Here's how the part is built. I have some questions about the finished solid (model axes, mm). Face numbers are marked on the shaded views. A direction names the side the tool comes from. Round coordinates to 2 decimals unless told otherwise and drop trailing zeros. Loops run counter-clockwise (first coordinate to the right, second up) from the corner with the lowest first, then second, coordinate; pieces in that order, holes last. Notation, with made-up numbers: M -16.5,54.5 L -6.5,54.5 A26 ccw -6.5,92.5 Z; hole C 82.25,50.25 d2. An arc over 180 degrees is marked long. Answer as a JSON object with one key per item and string values.
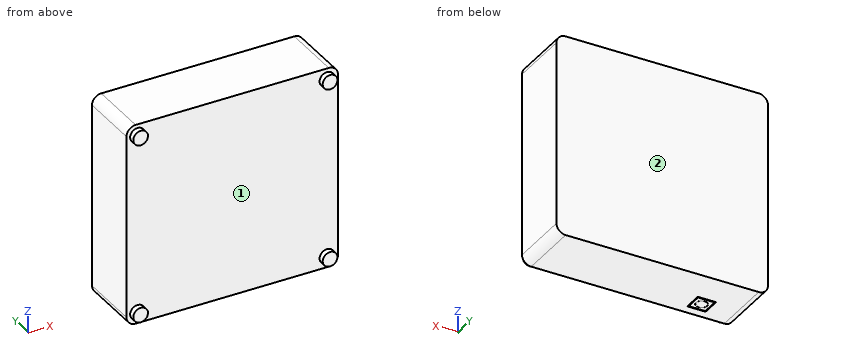
from build123d import *

# Parameters (mm, degrees)
EXTRUDE_1_DEPTH     = 33
SKETCH_2_R          = 4
EXTRUDE_2_DEPTH     = 3
SKETCH_3_W          = 10
SKETCH_3_H          = 10
SKETCH_3_W_2        = 9
SKETCH_3_H_2        = 9
CUT_EXTRUDE_1_DEPTH = 5
SKETCH_4_R          = 3.1
SKETCH_4_R_2        = 3
CUT_EXTRUDE_2_DEPTH = 10


with BuildPart() as part:
    # 草图1 → 凸台-拉伸1 (new body)
    with BuildSketch(Plane(origin=(0, 0, 0), x_dir=(1, 0, 0), z_dir=(0, 1, 0))):
        with BuildLine():
            Line((-52.5, 55), (52.5, 55))
            ThreePointArc((52.5, 55), (56.035533906, 53.535533906), (57.5, 50))
            Line((57.5, 50), (57.5, -50))
            ThreePointArc((57.5, -50), (56.035533906, -53.535533906), (52.5, -55))
            Line((52.5, -55), (-52.5, -55))
            ThreePointArc((-52.5, -55), (-56.035533906, -53.535533906), (-57.5, -50))
            Line((-57.5, -50), (-57.5, 50))
            ThreePointArc((-57.5, 50), (-56.035533906, 53.535533906), (-52.5, 55))
        make_face()
    extrude(amount=EXTRUDE_1_DEPTH)

    # 草图2 → 凸台-拉伸2 (add)
    with BuildSketch(Plane.XZ):
        with Locations(Location((-51.5, 49, 0), (0, 0, 270))):
            Circle(SKETCH_2_R)
        with Locations(Location((51.5, 49, 0), (0, 0, 270))):
            Circle(SKETCH_2_R)
        with Locations(Location((-51.5, -49, 0), (0, 0, 270))):
            Circle(SKETCH_2_R)
        with Locations(Location((51.5, -49, 0), (0, 0, 270))):
            Circle(SKETCH_2_R)
    extrude(amount=EXTRUDE_2_DEPTH)

    # 草图3 → 切除-拉伸1 (cut)
    with BuildSketch(Plane(origin=(0, 0, -55), x_dir=(-1, 0, 0), z_dir=(0, 0, -1))):
        with Locations((34.5, 10)):
            Rectangle(SKETCH_3_W, SKETCH_3_H)
        with Locations((34.5, 10)):
            Rectangle(SKETCH_3_W_2, SKETCH_3_H_2, mode=Mode.SUBTRACT)
    extrude(amount=-CUT_EXTRUDE_1_DEPTH, mode=Mode.SUBTRACT)

    # 草图4 → 切除-拉伸2 (cut)
    with BuildSketch(Plane(origin=(0, 0, -55), x_dir=(-1, 0, 0), z_dir=(0, 0, -1))):
        with Locations((34.5, 10)):
            Circle(SKETCH_4_R)
        with Locations((34.5, 10)):
            Circle(SKETCH_4_R_2, mode=Mode.SUBTRACT)
    extrude(amount=-CUT_EXTRUDE_2_DEPTH, mode=Mode.SUBTRACT)


solid = part.part
Item 1: If I drill on L1, parallel to Y at x = -9.5, z = -45, over which ranges is the centre line in solid material (lowest first)? Write a range as from..to.
Solution:
{"L1": "y = 0..33"}
Item 2: I want a section at C-C on x = 19.5. List the corners of the cut face in (y, z) for me, plus the area to 3 significant figures.
Solution:
{"outline": "M 0,-55 L 33,-55 L 33,55 L 0,55 Z", "area": "3,630 mm2"}
Item 3: I want a section at A-A on x = -34.5. List the corners of the cut face in (y, z) for me.
Solution:
{"outline": "M 0,-55 L 5,-55 L 5,-50 L 5.5,-50 L 5.5,-55 L 6.9,-55 L 6.9,-45 L 7,-45 L 7,-55 L 13,-55 L 13,-45 L 13.1,-45 L 13.1,-55 L 14.5,-55 L 14.5,-50 L 15,-50 L 15,-55 L 33,-55 L 33,55 L 0,55 Z"}
Item 4: I want a section at B-B on z = -22.5. List the corners of the cut face in (x, y) for me.
Solution:
{"outline": "M -57.5,0 L 57.5,0 L 57.5,33 L -57.5,33 Z"}
Item 5: For P1, Ø2.5, axis at y = 10, z = -52.5, coming from the +X side; P2, Ø1.5, axis at x = -34, z = -51.5, coming from the -Y side; P3, Ø2.5, axis at y = 12, z = -52, coming from the -X side, each with a flat end and sliding along its axis, tell me the tip position at first contact or that it passes through.
Solution:
{"P1": "stops at x = 57.34", "P2": "stops at y = 0", "P3": "stops at x = -57.44"}
Item 6: For the marked faces 1 and 2, which set-ups out of +Z, -Z, +X, -X, +Y, -Y let a thin tool reach every point of the face, with its end or its side?
Solution:
{"face 1": "-Y", "face 2": "+Z, -Z, +X, -X, +Y"}
